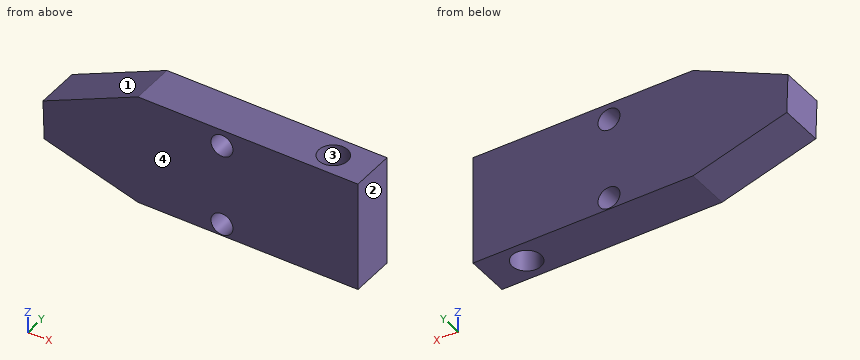
```python
from build123d import *

# Parameters (mm, degrees)
F0_W     = 25
F0_H     = 25
F1_DEPTH = 10
F3_D     = 5
F4_W     = 10
F4_H     = 25
F5_DEPTH = 25
F6_R     = 3.281956
F7_DEPTH = 25


with BuildPart() as f1:
    # F0 (on Front) → F1 (new body)
    with BuildSketch(Plane.XZ):
        Polygon((-11.585821, -12.109886), (-11.585821, 12.890114), (-33.171643, 3.001011), (-32.910448, -5.879586), align=None)
        with Locations((0.914179, 0.390114)):
            Rectangle(F0_W, F0_H)
    extrude(amount=F1_DEPTH)

    # F3 (through all)
    with Locations(Plane.XZ.offset(10)):
        with Locations((7.505033, 9.196309), (7.505033, -9.407719)):
            Hole(F3_D / 2)

    # F4 (on face) → F5 (join)
    with BuildSketch(Plane.YZ.offset(13.414179)):
        with Locations((-5, 0.390114)):
            Rectangle(F4_W, F4_H)
    extrude(amount=F5_DEPTH)

    # F6 (on face) → F7 (cut)
    with BuildSketch(Plane.XY.offset(12.890114)):
        with Locations((29.491611, -4.968121)):
            Circle(F6_R)
    extrude(amount=-F7_DEPTH, mode=Mode.SUBTRACT)


solid = f1.part
```
Geometry check sheet. Reference: the model listing, model coordinates, mm. Face numbers are marked on the shaded views. Round coordinates to 2 decimals unless told otherwise and drop trailing zeros. Write each loop counter-clockwise with the first axis right and the second up, starting at its lowest first coordinate (ties: lowest second). Pieces come first, ordered by that corner, then holes. Notation, with made-up numbers: (44, 76) - (88, 76) arc R26 ccw to (88, 106) - close; hole circle Ø6 at (53.5, 68.5). An arc over 180 degrees is marked (long way). Write each question's results on one line, items separated by ' | '.
(1) Depth check by flat-ended pin: pin 1 Ø6 at (x, y) = (29.49, -4.97) entering from -Z. Enter the tip coordinate at first touch or a pass-through.
Computed:
pin 1: passes through
(2) Sectioned sample at A-A, the plane z = 11. Enter the section's corners in (x, y).
Computed:
outline: (-15.71, -10) - (5.77, -10) - (5.77, 0) - (-15.71, 0) - close; (9.24, -10) - (38.41, -10) - (38.41, 0) - (9.24, 0) - close; hole circle Ø6.56 at (29.49, -4.97)
(3) Draft check along X on the marked faces 1, 2, 3 and 4. Enter one of: pulls with the +X half, pulls with the -X half, needs draft (parallel to the pull), parting line crosses it, or undercut.
Computed:
face 1: pulls with the -X half | face 2: pulls with the +X half | face 3: undercut | face 4: needs draft
(4) Sectioned sample at C-C, the plane x = 9. Enter the section's corners in (y, z).
Computed:
outline: (-10, -12.11) - (0, -12.11) - (0, -11.41) - (-10, -11.41) - close; (-10, -7.4) - (0, -7.4) - (0, 7.19) - (-10, 7.19) - close; (-10, 11.2) - (0, 11.2) - (0, 12.89) - (-10, 12.89) - close
(5) Sectioned sample at B-B, the plane y = -7.25. Enter the section's corners in (x, z), plus the area to 3 significant figures.
Computed:
outline: (-33.17, 3) - (-32.91, -5.88) - (-11.59, -12.11) - (27.13, -12.11) - (27.13, 12.89) - (-11.59, 12.89) - close; (31.85, -12.11) - (38.41, -12.11) - (38.41, 12.89) - (31.85, 12.89) - close; hole circle Ø5 at (7.51, -9.41); hole circle Ø5 at (7.51, 9.2) | area: 1,460 mm^2
(6) Thickness scan on probe 1 along X at (y, z) = (-3, 7.25); probe 2 along Z at (x, y) = (8, -1); probe 3 along X at (y, z) = (-8.75, 7). Record the ranges inside material, lowest first. Write a range as from..to.
Computed:
probe 1: x = -23.9..5.94, 9.07..26.87, 32.12..38.41 | probe 2: z = -12.11..-11.86, -6.96..6.75, 11.65..12.89 | probe 3: x = -24.44..6.31, 8.7..38.41
(7) Sectioned sample at D-D, the plane x = 29.5. Enter the section's corners in (y, z), plus the area to 3 significant figures.
Computed:
outline: (-10, -12.11) - (-8.25, -12.11) - (-8.25, 12.89) - (-10, 12.89) - close; (-1.69, -12.11) - (0, -12.11) - (0, 12.89) - (-1.69, 12.89) - close | area: 85.9 mm^2
